```python
from build123d import *

# Parameters (mm, degrees)
F0_W     = 25.4
F0_H     = 25.4
F1_DEPTH = 12.7
F3_DEPTH = 25.401
F4_R     = 1.78435
F5_DEPTH = 12.701


with BuildPart() as f1:
    # F0 (on Front) → F1 (new body)
    with BuildSketch(Plane.XZ):
        Rectangle(F0_W, F0_H)
    extrude(amount=F1_DEPTH)

    # F2 (on face) → F3 (cut, through all)
    with BuildSketch(Plane.XY.offset(12.7)):
        with BuildLine():
            ThreePointArc((-7.9375, 0), (0, -7.9375), (7.9375, 0))
            Line((7.9375, 0), (-7.9375, 0))
        make_face()
        with BuildLine():
            Line((-7.9375, 0), (7.9375, 0))
            ThreePointArc((7.9375, 0), (0, 7.9375), (-7.9375, 0))
        make_face()
    extrude(amount=-F3_DEPTH, mode=Mode.SUBTRACT)

    # F4 (on Front) → F5 (cut, through all)
    with BuildSketch(Plane.XZ):
        with Locations((-10.31748, 10.31748)):
            Circle(F4_R)
        with Locations((-10.31748, -10.31748)):
            Circle(F4_R)
        with Locations((10.31748, -10.31748)):
            Circle(F4_R)
        with Locations((10.31748, 10.31748)):
            Circle(F4_R)
    extrude(amount=F5_DEPTH, mode=Mode.SUBTRACT)


solid = f1.part
```
Could you check a few things on this model? Use its own coordinates, in mm. Round coordinates to 2 decimals unless told otherwise and drop trailing zeros. Loops run counter-clockwise (first coordinate to the right, second up) from the corner with the lowest first, then second, coordinate; pieces in that order, holes last. Notation, with made-up numbers: M 13.25,-11 L 39.25,-11 A18 ccw 39.25,-1 Z; hole C -35,40.25 d5. An arc over 180 degrees is marked long. Answer as CSV lines item,"result".
1) Imagine slicing it at D-D on y = -11.5. List the corners of the cut face in (x, z) for me.
From the geometry:
outline,"M -12.7,-12.7 L 12.7,-12.7 L 12.7,12.7 L -12.7,12.7 Z; hole C -10.32,-10.32 d3.57; hole C -10.32,10.32 d3.57; hole C 10.32,-10.32 d3.57; hole C 10.32,10.32 d3.57"
2) For pin 1 Ø3 at (x, z) = (-10.32, 10.32) entering from +Y; pin 2 Ø4 at (x, z) = (1.5, 7) entering from +Y, each with a flat end and sliding along its axis, tell me the tip position at first contact or that it passes through.
From the geometry:
pin 1,"through"
pin 2,"y = -7.12"
3) Imagine slicing it at B-B on y = -5.25. List the corners of the cut face in (x, z) for me, and give its area (3 significant figures).
From the geometry:
outline,"M -12.7,-12.7 L -5.95,-12.7 L -5.95,12.7 L -12.7,12.7 Z; M 5.95,-12.7 L 12.7,-12.7 L 12.7,12.7 L 5.95,12.7 Z; hole C -10.32,-10.32 d3.57; hole C -10.32,10.32 d3.57; hole C 10.32,-10.32 d3.57; hole C 10.32,10.32 d3.57"
area,"303 mm^2"
4) We'd pull the mould along X, two halves only. Please class faces 1 (the cylindrical face through (9, -6.26, 11.52)), 2 (the flat face through (10, 0, 0)), 3 (the cylindrical face through (-9.358, -6.261, 11.822)), 4 (the flat face through (-12.7, -6, 0)): released by +X, released by -X, zero draft, split by the parting line, or undercut.
From the geometry:
face 1,"undercut"
face 2,"zero draft"
face 3,"undercut"
face 4,"released by -X"
5) Imagine slicing it at A-A on x = -9. List the corners of the cut face in (y, z) for me, and give its area (3 significant figures).
From the geometry:
outline,"M -12.7,-12.7 L 0,-12.7 L 0,-11.52 L -12.7,-11.52 Z; M -12.7,-9.11 L 0,-9.11 L 0,9.11 L -12.7,9.11 Z; M -12.7,11.52 L 0,11.52 L 0,12.7 L -12.7,12.7 Z"
area,"261 mm^2"
6) If I drill on probe 1 along X at (y, z) = (-3.5, -10.5); probe 2 along X at (y, z) = (-7.25, -10.5); probe 3 along X at (y, z) = (-0.25, 7.5), over which ranges is the centre line in solid material (lowest first)?
From the geometry:
probe 1,"-12.7 to -12.09, -8.54 to -7.12, 7.12 to 8.54, 12.09 to 12.7"
probe 2,"-12.7 to -12.09, -8.54 to -3.23, 3.23 to 8.54, 12.09 to 12.7"
probe 3,"-12.7 to -7.93, 7.93 to 12.7"
7) Imagine slicing it at C-C on z = -10. List the corners of the cut face in (x, y) for me (1 decimal), and give its area (3 significant figures).
From the geometry:
outline,"M -12.7,-12.7 L -12.1,-12.7 L -12.1,0 L -12.7,0 Z; M -8.6,-12.7 L 8.6,-12.7 L 8.6,0 L 7.9,0 A7.9 cw -7.9,0 L -8.6,0 Z; M 12.1,-12.7 L 12.7,-12.7 L 12.7,0 L 12.1,0 Z"
area,"134 mm^2"
